from build123d import *

# Parameters (mm, degrees)
ESQUISSE1_R        = 1.1
ESQUISSE1_R_2      = 1.5
ESQUISSE1_R_3      = 2.5
BOSS_EXTRU_1_DEPTH = 5
BOSS_EXTRU_2_DEPTH = 20


with BuildPart() as part:
    # Esquisse1 → Boss.-Extru.1 (new body)
    with BuildSketch(Plane.XY):
        with BuildLine():
            Line((5.726385479, 8.801051605), (-30.755113053, 32.537660912))
            ThreePointArc((-30.755113053, 32.537660912), (-41.910189263, 31.619393351), (-39.730753447, 20.640823312))
            Line((-39.730753447, 20.640823312), (-6.890823906, -7.922534058))
            ThreePointArc((-6.890823906, -7.922534058), (8.382037853, -6.32387867), (5.726385479, 8.801051605))
        make_face()
        with Locations((0, 8)):
            Circle(ESQUISSE1_R, mode=Mode.SUBTRACT)
        with Locations((8, 0)):
            Circle(ESQUISSE1_R, mode=Mode.SUBTRACT)
        with Locations((0, -8)):
            Circle(ESQUISSE1_R, mode=Mode.SUBTRACT)
        with Locations((-8, 0)):
            Circle(ESQUISSE1_R, mode=Mode.SUBTRACT)
        with Locations((-35.923019369, 27.102337158)):
            Circle(ESQUISSE1_R_2, mode=Mode.SUBTRACT)
        Circle(ESQUISSE1_R_3, mode=Mode.SUBTRACT)
    boss_extru_1 = extrude(amount=BOSS_EXTRU_1_DEPTH)

    # Esquisse2 → Boss.-Extru.2 (add)
    with BuildSketch(Plane(origin=(0, 0, 0), x_dir=(-1, 0, 0), z_dir=(0, 0, -1))):
        Polygon((17.847870487, 24.139591031), (28.111906813, 10.535038273), (31.893676134, 13.824327565), (22.048994358, 26.873043329), align=None)
    boss_extru_2 = extrude(amount=BOSS_EXTRU_2_DEPTH)

    # Symétrie1: Boss.-Extru.1, Boss.-Extru.2 across plane
    add(boss_extru_1.mirror(Plane.XY.offset(-20)))
    add(boss_extru_2.mirror(Plane.XY.offset(-20)))


solid = part.part
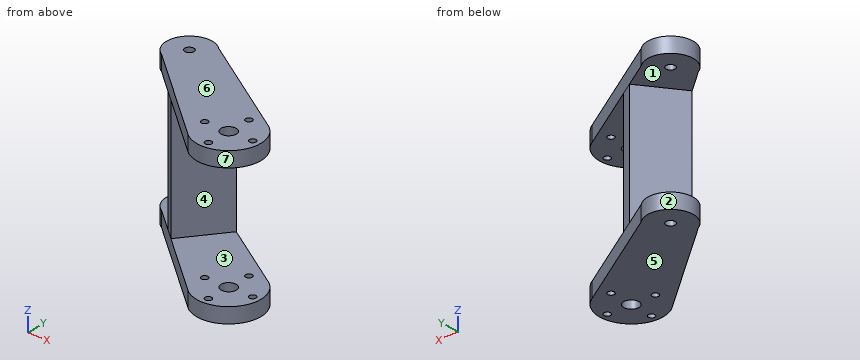
Part model, mm, in its own coordinate system. Face numbers are marked on the shaded views. A direction names the side the tool comes from. Coordinates: 2 decimals unless noted, no trailing zeros. Write each loop counter-clockwise with the first axis right and the second up, starting at its lowest first coordinate (ties: lowest second). Pieces come first, ordered by that corner, then holes. Notation, with made-up numbers: M -35,81 L 22,81 A25 cw 22,120 Z; hole C 11,65 d3. An arc over 180 degrees is marked long. Return JSON: item names as keys, results as strings.
1. Probe L1, parallel to Z at x = -3.5, y = 14; L2, parallel to Y at x = 0, z = -41; L3, parallel to Y at x = -22, z = -27.5. List the from-to ranges inside material, lowest first.
Determined:
{"L1": "-45 to -40, 0 to 5", "L2": "-10.5 to -9.1, -6.9 to -2.5, 2.5 to 6.9, 9.1 to 12.53", "L3": "18.64 to 26.84"}
2. Saw through at B-B, the plane y = -5.5. Write the cut outline in (x, z).
Determined:
{"outline": "M -9.68,-45 L 8.94,-45 L 8.94,-40 L -9.68,-40 Z; M -9.68,0 L 8.94,0 L 8.94,5 L -9.68,5 Z"}
3. Saw through at A-A, the plane x = -8. Write the cut outline in (y, z), then the cut area to 3 significant figures.
Determined:
{"outline": "M -6.96,-45 L -1.1,-45 L -1.1,-40 L -6.96,-40 Z; M -6.96,0 L -1.1,0 L -1.1,5 L -6.96,5 Z; M 1.1,-45 L 17.73,-45 L 17.73,-40 L 1.1,-40 Z; M 1.1,0 L 17.73,0 L 17.73,5 L 1.1,5 Z", "area": "225 mm²"}
4. 3-axis set-ups, long thin cutter, end or side, ignore diameter. For the marked faces 1, 2 and 3: which of +Z, -Z, +X, -X, +Y, -Y reach the whole face in a straight line?
Determined:
{"face 1": "-X, +Y", "face 2": "+Z, -Z", "face 3": "+X, -Y"}
5. Flat gauge pins, fed straight in: pin 1 Ø2 at (x, y) = (8, 0) entering from +Z; pin 2 Ø6 at (x, z) = (-14, -2.5) entering from -Y; pin 3 Ø10 at (y, z) = (9.5, -1) entering from -X. Where does each tip first touch, or does it go through?
Determined:
{"pin 1": "through", "pin 2": "y = -3.18", "pin 3": "x = -32.55"}
6. Saw through at C-C, the plane y = 8. Write the cut outline in (x, z).
Determined:
{"outline": "M -25.2,-45 L -1.1,-45 L -1.1,-40 L -25.2,-40 Z; M -25.2,0 L -1.1,0 L -1.1,5 L -25.2,5 Z; M 1.1,-45 L 6.8,-45 L 6.8,-40 L 1.1,-40 Z; M 1.1,0 L 6.8,0 L 6.8,5 L 1.1,5 Z"}
7. Pull direction Z, two halves, no side cores. Call the marked faces 4, 5, 6 and 7: pulls with the +Z half, pulls with the -Z half, needs draft (parallel to the pull), parting line crosses it, or undercut.
Determined:
{"face 4": "undercut", "face 5": "pulls with the -Z half", "face 6": "pulls with the +Z half", "face 7": "needs draft"}
8. Saw through at D-D, the plane y = 0. Count the separate pieces of the cut face and the enclosed holes in it, then the cut area to 3 significant figures.
Determined:
{"separate pieces": "8", "enclosed holes": "0", "area": "171 mm²"}
